```python
from build123d import *

# Parameters (mm, degrees)
SKETCH1_R            = 65
BOSS_EXTRUDE1_DEPTH  = 5
BOSS_EXTRUDE2_DEPTH  = 50
BOSS_EXTRUDE3_DEPTH  = 45
BOSS_EXTRUDE4_DEPTH  = 45
BOSS_EXTRUDE6_DEPTH  = 45
BOSS_EXTRUDE7_DEPTH  = 45
BOSS_EXTRUDE9_DEPTH  = 45
BOSS_EXTRUDE10_DEPTH = 45
SKETCH11_R           = 4.25
CUT_EXTRUDE1_DEPTH   = 10


with BuildPart() as part:
    # Sketch1 → Boss-Extrude1 (new body)
    with BuildSketch(Plane.XY.offset(5)):
        Circle(SKETCH1_R)
    extrude(amount=-BOSS_EXTRUDE1_DEPTH)

    # Sketch2 → Boss-Extrude2 (add)
    with BuildSketch(Plane.XY.offset(5)):
        with BuildLine():
            Line((-2.896618782, -15.740746549), (-2.896618782, -22.312767637))
            ThreePointArc((-2.896618782, -22.312767637), (-19.472098251, -11.273304294), (-20.792365892, 8.598111457))
            Line((-20.792365892, 8.598111457), (-15.098298122, 5.310639897))
            ThreePointArc((-15.098298122, 5.310639897), (-13.847182977, -8.026021796), (-2.896618782, -15.740746549))
        make_face()
        with BuildLine():
            Line((17.842365892, 13.707661339), (12.148298122, 10.420189779))
            ThreePointArc((12.148298122, 10.420189779), (-0.027147278, 16.005023127), (-12.183576995, 10.378918724))
            Line((-12.183576995, 10.378918724), (-17.875114212, 13.664929269))
            ThreePointArc((-17.875114212, 13.664929269), (-0.026918777, 22.499983897), (17.842365892, 13.707661339))
        make_face()
        with BuildLine():
            Line((2.95, -22.305772795), (2.95, -15.730829675))
            ThreePointArc((2.95, -15.730829675), (13.874330255, -7.979001331), (15.080195777, 5.361827824))
            Line((15.080195777, 5.361827824), (20.771732993, 8.647838368))
            ThreePointArc((20.771732993, 8.647838368), (19.499017028, -11.226679604), (2.95, -22.305772795))
        make_face()
    extrude(amount=BOSS_EXTRUDE2_DEPTH)

    # Sketch3 → Boss-Extrude3 (add)
    with BuildSketch(Plane.XY.offset(5)):
        with BuildLine():
            Line((-33.850308879, 16.137118355), (-20.792365892, 8.598111457))
            ThreePointArc((-20.792365892, 8.598111457), (-21.975466771, 4.82999588), (-22.481466179, 0.913059924))
            Line((-22.481466179, 0.913059924), (-36.414511458, 8.957307367))
            ThreePointArc((-36.414511458, 8.957307367), (-35.315346037, 12.612546701), (-33.850308879, 16.137118355))
        make_face()
    extrude(amount=BOSS_EXTRUDE3_DEPTH)

    # Sketch4 → Boss-Extrude4 (add)
    with BuildSketch(Plane.XY.offset(5)):
        with BuildLine():
            Line((-10.45, -36.014545673), (-10.45, -19.926050788))
            ThreePointArc((-10.45, -19.926050788), (-6.804834253, -21.446310424), (-2.95, -22.305772795))
            Line((-2.95, -22.305772795), (-2.95, -37.383786593))
            ThreePointArc((-2.95, -37.383786593), (-6.734887169, -36.890260162), (-10.45, -36.014545673))
        make_face()
    extrude(amount=BOSS_EXTRUDE4_DEPTH)

    # Sketch6 → Boss-Extrude6 (add)
    with BuildSketch(Plane.XY.offset(5)):
        with BuildLine():
            Line((30.900308879, 21.246668237), (17.842365892, 13.707661339))
            ThreePointArc((17.842365892, 13.707661339), (15.170632518, 16.616314543), (12.031466179, 19.012990863))
            Line((12.031466179, 19.012990863), (25.964511458, 27.057238306))
            ThreePointArc((25.964511458, 27.057238306), (28.580458868, 24.277713461), (30.900308879, 21.246668237))
        make_face()
    extrude(amount=BOSS_EXTRUDE6_DEPTH)

    # Sketch7 → Boss-Extrude7 (add)
    with BuildSketch(Plane.XY.offset(5)):
        with BuildLine():
            Line((-25.964511458, 27.057238306), (-12.031466179, 19.012990863))
            ThreePointArc((-12.031466179, 19.012990863), (-15.170632518, 16.616314543), (-17.842365892, 13.707661339))
            Line((-17.842365892, 13.707661339), (-30.900308879, 21.246668237))
            ThreePointArc((-30.900308879, 21.246668237), (-28.580458868, 24.277713461), (-25.964511458, 27.057238306))
        make_face()
    extrude(amount=BOSS_EXTRUDE7_DEPTH)

    # Sketch9 → Boss-Extrude9 (add)
    with BuildSketch(Plane.XY.offset(5)):
        with BuildLine():
            Line((2.95, -37.383786593), (2.95, -22.305772795))
            ThreePointArc((2.95, -22.305772795), (6.804834253, -21.446310424), (10.45, -19.926050788))
            Line((10.45, -19.926050788), (10.45, -36.014545673))
            ThreePointArc((10.45, -36.014545673), (6.734887169, -36.890260162), (2.95, -37.383786593))
        make_face()
    extrude(amount=BOSS_EXTRUDE9_DEPTH)

    # Sketch10 → Boss-Extrude10 (add)
    with BuildSketch(Plane.XY.offset(5)):
        with BuildLine():
            Line((36.414511458, 8.957307367), (22.481466179, 0.913059924))
            ThreePointArc((22.481466179, 0.913059924), (21.975466771, 4.82999588), (20.792365892, 8.598111457))
            Line((20.792365892, 8.598111457), (33.850308879, 16.137118355))
            ThreePointArc((33.850308879, 16.137118355), (35.315346037, 12.612546701), (36.414511458, 8.957307367))
        make_face()
    extrude(amount=BOSS_EXTRUDE10_DEPTH)

    # Sketch11 → Cut-Extrude1 (cut)
    with BuildSketch(Plane.XY.offset(5)):
        with Locations((-25, 45)):
            Circle(SKETCH11_R)
        with Locations((25, 45)):
            Circle(SKETCH11_R)
        with Locations((26.47114317, -44.150635095)):
            Circle(SKETCH11_R)
        with Locations((51.47114317, -0.849364905)):
            Circle(SKETCH11_R)
        with Locations((-51.47114317, -0.849364905)):
            Circle(SKETCH11_R)
        with Locations((-26.47114317, -44.150635095)):
            Circle(SKETCH11_R)
    extrude(amount=-CUT_EXTRUDE1_DEPTH, mode=Mode.SUBTRACT)


solid = part.part
```
Geometry check sheet. Reference: the model listing, model coordinates, mm. A direction names the side the tool comes from. Coordinates: 2 decimals unless noted, no trailing zeros. Loops run counter-clockwise (first coordinate to the right, second up) from the corner with the lowest first, then second, coordinate; pieces in that order, holes last. Notation, with made-up numbers: (21.25, -16.5) - (31.25, -16.5) arc R13 ccw to (31.25, -2.5) - close; hole circle Ø7 at (-24, -15.5). An arc over 180 degrees is marked (long way). One line per item, written item: value. Start each with the question number.
(1) Cross-section at A-A on z = 44.5. Count the separate pieces of the cut face and the enclosed holes in it, plus the area to 3 significant figures.
(2) Material ranges on line 1 (Z direction, x = 48, y = -7); line 2 (X direction, y = -28.5, z = 28); line 3 (X direction, y = -1, z = 43), recorded low to high. Write a range as [from, to].
(3) Mould release check, pull along X, two halves, no side actions. Record for faces 1 (the flat face through (-2.95, -30, 27)), 2 (the flat face through (7, -29, 50)), 3 (the cylindrical face through (-28.615, 24.237, 27.185)): released by +X, released by -X, zero draft, split by the parting line, or undercut.
(4) Cross-section at B-B on x = 0. Enter the section's corners in (y, z).
(5) Tool access check on faces 4 (the flat face through (18.9, 22.98, 27.18)), 5 (the flat face through (2.95, -27, 30)), 6 (the flat face through (10.45, -28, 27)). Record the directions out of +Z, -Z, +X, -X, +Y, -Y that give a thin tool (end or side, any length) a straight path to the whole face; none if there is none.
(6) Depth check by flat-ended pin: P1, Ø13.5, axis at x = -26.47, y = -44.15, coming from the +Z side; P2, Ø16.5, axis at x = -31.5, y = 7.5, coming from the +Z side; P3, Ø5, axis at x = -12.5, z = 27, coming from the +Y side; P4, Ø7.5, axis at x = -51.47, y = -0.85, coming from the -Z side. Enter the tip coordinate at first touch or a pass-through.
Results below:
1. separate pieces: 3
1. enclosed holes: 0
1. area: 1,370 mm2
2. line 1: z = [0, 5]
2. line 2: x = [-10.45, -2.95], [2.95, 10.45]
2. line 3: x = [-22.48, -15.97], [15.97, 22.48]
3. face 1: undercut
3. face 2: zero draft
3. face 3: released by -X
4. outline: (-65, 0) - (65, 0) - (65, 5) - (22.5, 5) - (22.5, 55) - (16.01, 55) - (16.01, 5) - (-65, 5) - close
5. face 4: +Z, +Y
5. face 5: +Z, -Y
5. face 6: +Z, +X, -Y
6. P1: stops at z = 5
6. P2: stops at z = 50
6. P3: stops at y = 20.73
6. P4: passes through
